Can you work these out from the model? Positions are in its coordinate system, mm. Face numbers are marked on the shaded views. A direction names the side the tool comes from. Coordinates: 2 decimals unless noted, no trailing zeros. Order: outer loops, then holes, each group sorted by start corner. A loop starts at its lowest first (then second) coordinate and runs counter-clockwise, first axis right, second up. Notation, with made-up numbers: (10, 25) - (65, 25) arc R23 ccw to (65, 60) - close; hole circle Ø11 at (20.25, -12). An arc over 180 degrees is marked (long way). Use a Markdown table: item, result. Add a question column.
(1) I want a section at A-A (z = 39.5). List the corners of the cut face in (x, y) for me.
(2) I want a section at D-D (y = -18.5). List the corners of the cut face in (x, z) for me, and give its area (3 significant figures).
(3) On a 3-axis mill with a long thin cutter (end or side, diameter ignored), from which of +Z, -Z, +X, -X, +Y, -Y can I reach the whole of each face in a straight line? I mean the marked faces 1, 2 and 3. Say none if no direction works.
(4) We'd pull the mould along X, two halves only. Please class the marked faces 4, 5 and 6: pulls with the +X half, pulls with the -X half, needs draft (parallel to the pull), parting line crosses it, or undercut.
(5) For pin 1 Ø20.5 at (x, z) = (-18, 30) entering from -Y; pin 2 Ø10.5 at (y, z) = (-21.745, 18.725) entering from +X; pin 3 Ø2 at (x, y) = (-13.5, -5.25) entering from -Z; pin 4 Ø0.6 at (x, y) = (4.5, -25.5) entering from +Z, each with a flat end and sliding along its axis, tell me the tip position at first contact or that it passes through.
(6) If I drill on L1, parallel to X at y = -5.25, z = 2.75; L2, parallel to Y at x = -1.1, z = 6; L3, parallel to X at y = -11.5, z = 17.5, over which ranges is the centre line in solid material (lowest first)? Write a range as [from, to].
(7) I want a section at C-C (x = -17). List the corners of the cut face in (y, z) for me, and give its area (3 significant figures).
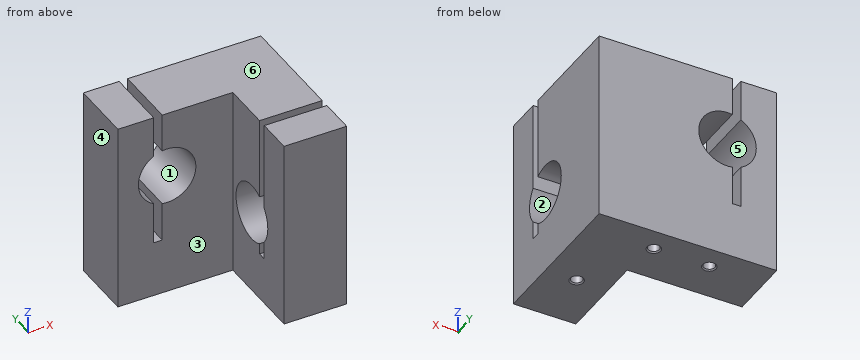
```python
from build123d import *

# Parameters (mm, degrees)
SKETCH1_W                       = 25.65
SKETCH1_H                       = 14
SKETCH1_W_2                     = 14
SKETCH1_H_2                     = 34.73
BOSS_EXTRUDE1_DEPTH             = 42.65
SKETCH2_R                       = 6.425
CUT_EXTRUDE1_DEPTH              = 42.65
SKETCH3_W                       = 1.9
SKETCH3_H                       = 30
CUT_EXTRUDE2_DEPTH              = 42.65
SKETCH4_R                       = 6.425
CUT_EXTRUDE3_DEPTH              = 42.65
SKETCH5_W                       = 32
SKETCH5_H                       = 1.9
CUT_EXTRUDE4_DEPTH              = 42.65
M3X0_5_TAPPED_HOLE1_D           = 2.5
M3X0_5_TAPPED_HOLE1_DEPTH       = 10
M3X0_5_TAPPED_HOLE1_CSINK_D     = 3.05
M3X0_5_TAPPED_HOLE1_CSINK_ANGLE = 90
M3X0_5_TAPPED_HOLE1_TIP         = 0.751075774


with BuildPart() as part:
    # Sketch1 → Boss-Extrude1 (new body)
    with BuildSketch(Plane.XY):
        with Locations((-12.825, -7)):
            Rectangle(SKETCH1_W, SKETCH1_H)
        with Locations((7, -17.365)):
            Rectangle(SKETCH1_W_2, SKETCH1_H_2)
    extrude(amount=BOSS_EXTRUDE1_DEPTH)

    # Sketch2 → Cut-Extrude1 (cut)
    with BuildSketch(Plane.XZ.offset(14)):
        with Locations((-14.665, 27.725)):
            Circle(SKETCH2_R)
    extrude(amount=-CUT_EXTRUDE1_DEPTH, mode=Mode.SUBTRACT)

    # Sketch3 → Cut-Extrude2 (cut)
    with BuildSketch(Plane.XZ.offset(14)):
        with Locations((-16.7, 27.65)):
            Rectangle(SKETCH3_W, SKETCH3_H)
    extrude(amount=-CUT_EXTRUDE2_DEPTH, mode=Mode.SUBTRACT)

    # Sketch4 → Cut-Extrude3 (cut)
    with BuildSketch(Plane.ZY):
        with Locations(Location((18.725, -21.745, 0), (0, 0, 270))):
            Circle(SKETCH4_R)
    extrude(amount=-CUT_EXTRUDE3_DEPTH, mode=Mode.SUBTRACT)

    # Sketch5 → Cut-Extrude4 (cut)
    with BuildSketch(Plane.ZY):
        with Locations((26.65, -25.78)):
            Rectangle(SKETCH5_W, SKETCH5_H)
    extrude(amount=-CUT_EXTRUDE4_DEPTH, mode=Mode.SUBTRACT)

    # M3x0.5 Tapped Hole1
    with Locations(Plane(origin=(0, 0, 0), x_dir=(-1, 0, 0), z_dir=(0, 0, -1))):
        with Locations((1.1, -5.25), (13.5, -5.25), (-6.99, -21.8)):
            CounterSinkHole(M3X0_5_TAPPED_HOLE1_D / 2, M3X0_5_TAPPED_HOLE1_CSINK_D / 2, depth=M3X0_5_TAPPED_HOLE1_DEPTH, counter_sink_angle=M3X0_5_TAPPED_HOLE1_CSINK_ANGLE)
            with Locations((0, 0, -(M3X0_5_TAPPED_HOLE1_DEPTH + M3X0_5_TAPPED_HOLE1_TIP / 2))):  # 118° drill point
                Cone(0, M3X0_5_TAPPED_HOLE1_D / 2, M3X0_5_TAPPED_HOLE1_TIP, mode=Mode.SUBTRACT)


solid = part.part
```
Answers follow:
| question | item | result |
|---|---|---|
| 1 | outline | (-25.65, -14) - (-17.65, -14) - (-17.65, 0) - (-25.65, 0) - close; (-15.75, -14) - (0, -14) - (0, -24.83) - (14, -24.83) - (14, 0) - (-15.75, 0) - close; (0, -34.73) - (14, -34.73) - (14, -26.73) - (0, -26.73) - close |
| 2 | outline | (0, 0) - (14, 0) - (14, 13.18) - (0, 13.18) - close; (0, 24.27) - (14, 24.27) - (14, 42.65) - (0, 42.65) - close |
| 2 | area | 442 mm² |
| 3 | face 1 | +Y, -Y |
| 3 | face 2 | +X, -X |
| 3 | face 3 | +Z, -Z, -X, -Y |
| 4 | face 4 | pulls with the -X half |
| 4 | face 5 | undercut |
| 4 | face 6 | needs draft |
| 5 | pin 1 | stops at y = -14 |
| 5 | pin 2 | passes through |
| 5 | pin 3 | stops at z = 10.15 |
| 5 | pin 4 | stops at z = 10.65 |
| 6 | L1 | x = [-25.65, -14.75], [-12.25, -2.35], [0.15, 14] |
| 6 | L2 | y = [-14, -6.5], [-4, 0] |
| 6 | L3 | x = [-25.65, -17.65], [-15.75, 14] |
| 7 | outline | (-14, 0) - (0, 0) - (0, 12.65) - (-14, 12.65) - close |
| 7 | area | 177 mm² |
